The model under review builds one solid part; all positions refer to its coordinate system, in mm. A direction names the side the tool comes from. Coordinates: 2 decimals unless noted, no trailing zeros. Order: outer loops, then holes, each group sorted by start corner. A loop starts at its lowest first (then second) coordinate and runs counter-clockwise, first axis right, second up. Notation, with made-up numbers: (-8, 23) -> (15, 23) arc R17 ccw to (15, 39) -> close; hole circle Ø7 at (54.25, 4). An arc over 180 degrees is marked (long way). Use CSV: the item, a comma, the result in double quotes. Start each with the question number.
```python
from build123d import *

# Parameters (mm, degrees)
SKETCH1_R           = 1.1
SKETCH1_R_2         = 1.099999998
SKETCH1_R_3         = 1.100000002
SKETCH1_R_4         = 1.100000004
SKETCH1_R_5         = 1.099999996
SKETCH1_R_6         = 1.5
BOSS_EXTRUDE1_DEPTH = 3
SKETCH2_W           = 6.5
SKETCH2_H           = 3.5
CUT_EXTRUDE1_DEPTH  = 3


with BuildPart() as part:
    # Sketch1 → Boss-Extrude1 (new body)
    with BuildSketch(Plane(origin=(0, 0, 0), x_dir=(1, 0, 0), z_dir=(0, 1, 0))):
        with BuildLine():
            Line((-65.541413555, 48.16007559), (-33.218669872, 45.046086874))
            ThreePointArc((-33.218669872, 45.046086874), (-32.739740879, 45.011528364), (-32.25970508, 45))
            Line((-32.25970508, 45), (32.25970508, 45))
            ThreePointArc((32.25970508, 45), (32.739740879, 45.011528364), (33.218669872, 45.046086874))
            Line((33.218669872, 45.046086874), (65.541413555, 48.16007559))
            ThreePointArc((65.541413555, 48.16007559), (68.051615849, 48.735029299), (70.331753828, 49.931966272))
            ThreePointArc((70.331753828, 49.931966272), (81.716587017, 44.695249474), (71.540883348, 37.381380156))
            ThreePointArc((71.540883348, 37.381380156), (69.074176187, 38.121003778), (66.500378347, 38.206162463))
            Line((66.500378347, 38.206162463), (37.020517604, 35.366058461))
            ThreePointArc((37.020517604, 35.366058461), (34.967820887, 34.700490182), (33.386772404, 33.231874971))
            ThreePointArc((33.386772404, 33.231874971), (34.463229219, 29.741424145), (35.835420758, 26.3562954))
            ThreePointArc((35.835420758, 26.3562954), (35.77253489, 25.409347753), (34.946904251, 24.941374967))
            ThreePointArc((34.946904251, 24.941374967), (33.213559493, 24.190832889), (32.5, 22.441938863))
            Line((32.5, 22.441938863), (32.5, -22.441938863))
            ThreePointArc((32.5, -22.441938863), (33.213559493, -24.190832889), (34.946904251, -24.941374967))
            ThreePointArc((34.946904251, -24.941374967), (35.77253489, -25.409347753), (35.835420758, -26.3562954))
            ThreePointArc((35.835420758, -26.3562954), (34.463229219, -29.741424145), (33.386772404, -33.231874971))
            ThreePointArc((33.386772404, -33.231874971), (34.967820887, -34.700490182), (37.020517604, -35.366058461))
            Line((37.020517604, -35.366058461), (66.500378347, -38.206162463))
            ThreePointArc((66.500378347, -38.206162463), (69.074176187, -38.121003778), (71.540883348, -37.381380156))
            ThreePointArc((71.540883348, -37.381380156), (81.716587017, -44.695249474), (70.331753828, -49.931966272))
            ThreePointArc((70.331753828, -49.931966272), (68.051615849, -48.735029299), (65.541413555, -48.16007559))
            Line((65.541413555, -48.16007559), (33.218669872, -45.046086874))
            ThreePointArc((33.218669872, -45.046086874), (32.739740879, -45.011528364), (32.25970508, -45))
            Line((32.25970508, -45), (-32.25970508, -45))
            ThreePointArc((-32.25970508, -45), (-32.739740879, -45.011528364), (-33.218669872, -45.046086874))
            Line((-33.218669872, -45.046086874), (-65.541413555, -48.16007559))
            ThreePointArc((-65.541413555, -48.16007559), (-68.051615849, -48.735029299), (-70.331753828, -49.931966272))
            ThreePointArc((-70.331753828, -49.931966272), (-81.716587017, -44.695249474), (-71.540883348, -37.381380156))
            ThreePointArc((-71.540883348, -37.381380156), (-69.074176187, -38.121003778), (-66.500378347, -38.206162463))
            Line((-66.500378347, -38.206162463), (-37.020517604, -35.366058461))
            ThreePointArc((-37.020517604, -35.366058461), (-34.967820887, -34.700490182), (-33.386772404, -33.231874971))
            ThreePointArc((-33.386772404, -33.231874971), (-34.463229219, -29.741424145), (-35.835420758, -26.3562954))
            ThreePointArc((-35.835420758, -26.3562954), (-35.77253489, -25.409347753), (-34.946904251, -24.941374967))
            ThreePointArc((-34.946904251, -24.941374967), (-33.213559493, -24.190832889), (-32.5, -22.441938863))
            Line((-32.5, -22.441938863), (-32.5, 22.441938863))
            ThreePointArc((-32.5, 22.441938863), (-33.213559493, 24.190832889), (-34.946904251, 24.941374967))
            ThreePointArc((-34.946904251, 24.941374967), (-35.77253489, 25.409347753), (-35.835420758, 26.3562954))
            ThreePointArc((-35.835420758, 26.3562954), (-34.463229219, 29.741424145), (-33.386772404, 33.231874971))
            ThreePointArc((-33.386772404, 33.231874971), (-34.967820887, 34.700490182), (-37.020517604, 35.366058461))
            Line((-37.020517604, 35.366058461), (-66.500378347, 38.206162463))
            ThreePointArc((-66.500378347, 38.206162463), (-69.074176187, 38.121003778), (-71.540883348, 37.381380156))
            ThreePointArc((-71.540883348, 37.381380156), (-81.716587017, 44.695249474), (-70.331753828, 49.931966272))
            ThreePointArc((-70.331753828, 49.931966272), (-68.051615849, 48.735029299), (-65.541413555, 48.16007559))
        make_face()
        with Locations(Location((-79, 44, 0), (0, 0, 270))):
            Circle(SKETCH1_R, mode=Mode.SUBTRACT)
        with Locations(Location((79, 44, 0), (0, 0, 270))):
            Circle(SKETCH1_R, mode=Mode.SUBTRACT)
        with Locations(Location((-74.500002544, 48.500002544, 0), (0, 0, 270))):
            Circle(SKETCH1_R_2, mode=Mode.SUBTRACT)
        with Locations(Location((-70, 44.000005089, 0), (0, 0, 270))):
            Circle(SKETCH1_R_3, mode=Mode.SUBTRACT)
        with Locations(Location((-74.499997456, 39.500002544, 0), (0, 0, 270))):
            Circle(SKETCH1_R_4, mode=Mode.SUBTRACT)
        with Locations(Location((-74.499997456, -39.500002544, 0), (0, 0, 270))):
            Circle(SKETCH1_R_3, mode=Mode.SUBTRACT)
        with Locations(Location((-70, -44.000005089, 0), (0, 0, 270))):
            Circle(SKETCH1_R_2, mode=Mode.SUBTRACT)
        with Locations(Location((-74.500002544, -48.500002544, 0), (0, 0, 270))):
            Circle(SKETCH1_R_5, mode=Mode.SUBTRACT)
        with Locations(Location((-79, -44, 0), (0, 0, 270))):
            Circle(SKETCH1_R, mode=Mode.SUBTRACT)
        with Locations(Location((79, -44, 0), (0, 0, 270))):
            Circle(SKETCH1_R, mode=Mode.SUBTRACT)
        with Locations(Location((74.500002544, -48.500002544, 0), (0, 0, 270))):
            Circle(SKETCH1_R_3, mode=Mode.SUBTRACT)
        with Locations(Location((70, -44.000005089, 0), (0, 0, 270))):
            Circle(SKETCH1_R_2, mode=Mode.SUBTRACT)
        with Locations(Location((74.499997456, -39.500002544, 0), (0, 0, 270))):
            Circle(SKETCH1_R_5, mode=Mode.SUBTRACT)
        with Locations(Location((74.499997456, 39.500002544, 0), (0, 0, 270))):
            Circle(SKETCH1_R_2, mode=Mode.SUBTRACT)
        with Locations(Location((70, 44.000005089, 0), (0, 0, 270))):
            Circle(SKETCH1_R_3, mode=Mode.SUBTRACT)
        with Locations(Location((74.500002544, 48.500002544, 0), (0, 0, 270))):
            Circle(SKETCH1_R_4, mode=Mode.SUBTRACT)
        with Locations(Location((-74.5, -44, 0), (0, 0, 270))):
            Circle(SKETCH1_R_6, mode=Mode.SUBTRACT)
        with Locations(Location((-74.5, 44, 0), (0, 0, 270))):
            Circle(SKETCH1_R_6, mode=Mode.SUBTRACT)
        with Locations(Location((74.5, 44, 0), (0, 0, 270))):
            Circle(SKETCH1_R_6, mode=Mode.SUBTRACT)
        with Locations(Location((74.5, -44, 0), (0, 0, 270))):
            Circle(SKETCH1_R_6, mode=Mode.SUBTRACT)
    extrude(amount=BOSS_EXTRUDE1_DEPTH)

    # Sketch2 → Cut-Extrude1 (cut)
    with BuildSketch(Plane(origin=(0, 3, 0), x_dir=(1, 0, 0), z_dir=(0, 1, 0))):
        with Locations((-17.75, 23.75)):
            Rectangle(SKETCH2_W, SKETCH2_H)
        with Locations((-17.75, -23.75)):
            Rectangle(SKETCH2_W, SKETCH2_H)
        with Locations((17.75, -23.75)):
            Rectangle(SKETCH2_W, SKETCH2_H)
        with Locations((17.75, 23.75)):
            Rectangle(SKETCH2_W, SKETCH2_H)
        with BuildLine():
            Line((-25.5, 19), (-4, 19))
            ThreePointArc((-4, 19), (-3.292893219, 18.707106781), (-3, 18))
            Line((-3, 18), (-3, 2.5))
            ThreePointArc((-3, 2.5), (-3.292893219, 1.792893219), (-4, 1.5))
            Line((-4, 1.5), (-25.5, 1.5))
            ThreePointArc((-25.5, 1.5), (-26.207106781, 1.792893219), (-26.5, 2.5))
            Line((-26.5, 2.5), (-26.5, 18))
            ThreePointArc((-26.5, 18), (-26.207106781, 18.707106781), (-25.5, 19))
        make_face()
        with BuildLine():
            Line((-25.5, -1.5), (-4, -1.5))
            ThreePointArc((-4, -1.5), (-3.292893219, -1.792893219), (-3, -2.5))
            Line((-3, -2.5), (-3, -18))
            ThreePointArc((-3, -18), (-3.292893219, -18.707106781), (-4, -19))
            Line((-4, -19), (-25.5, -19))
            ThreePointArc((-25.5, -19), (-26.207106781, -18.707106781), (-26.5, -18))
            Line((-26.5, -18), (-26.5, -2.5))
            ThreePointArc((-26.5, -2.5), (-26.207106781, -1.792893219), (-25.5, -1.5))
        make_face()
        with BuildLine():
            Line((4, 19), (25.5, 19))
            ThreePointArc((25.5, 19), (26.207106781, 18.707106781), (26.5, 18))
            Line((26.5, 18), (26.5, 2.5))
            ThreePointArc((26.5, 2.5), (26.207106781, 1.792893219), (25.5, 1.5))
            Line((25.5, 1.5), (4, 1.5))
            ThreePointArc((4, 1.5), (3.292893219, 1.792893219), (3, 2.5))
            Line((3, 2.5), (3, 18))
            ThreePointArc((3, 18), (3.292893219, 18.707106781), (4, 19))
        make_face()
        with BuildLine():
            Line((4, -1.5), (25.5, -1.5))
            ThreePointArc((25.5, -1.5), (26.207106781, -1.792893219), (26.5, -2.5))
            Line((26.5, -2.5), (26.5, -18))
            ThreePointArc((26.5, -18), (26.207106781, -18.707106781), (25.5, -19))
            Line((25.5, -19), (4, -19))
            ThreePointArc((4, -19), (3.292893219, -18.707106781), (3, -18))
            Line((3, -18), (3, -2.5))
            ThreePointArc((3, -2.5), (3.292893219, -1.792893219), (4, -1.5))
        make_face()
        with BuildLine():
            Line((-17.595187003, 39), (17.595187003, 39))
            ThreePointArc((17.595187003, 39), (18.554660419, 38.281799152), (18.135944594, 37.158821525))
            Line((18.135944594, 37.158821525), (0.540757591, 25.84762988))
            ThreePointArc((0.540757591, 25.84762988), (0, 25.688808356), (-0.540757591, 25.84762988))
            Line((-0.540757591, 25.84762988), (-18.135944594, 37.158821525))
            ThreePointArc((-18.135944594, 37.158821525), (-18.554660419, 38.281799152), (-17.595187003, 39))
        make_face()
        with BuildLine():
            Line((-17.595187003, -39), (17.595187003, -39))
            ThreePointArc((17.595187003, -39), (18.554660419, -38.281799152), (18.135944594, -37.158821525))
            Line((18.135944594, -37.158821525), (0.540757591, -25.84762988))
            ThreePointArc((0.540757591, -25.84762988), (0, -25.688808356), (-0.540757591, -25.84762988))
            Line((-0.540757591, -25.84762988), (-18.135944594, -37.158821525))
            ThreePointArc((-18.135944594, -37.158821525), (-18.554660419, -38.281799152), (-17.595187003, -39))
        make_face()
    extrude(amount=-CUT_EXTRUDE1_DEPTH, mode=Mode.SUBTRACT)


solid = part.part
```
Q1. Add section C-C, the plane y = 1.55. State how many separate pieces and enclosed holes the cut face has, then the cut area to 3 significant figures.
Q2. Add section D-D, the plane x = 30. State the section outline as (y, z) points, then the cut area to 3 significant figures.
Q3. Clearance check with flat-ended pins moving along their axes: pin 1 Ø0.9 at (x, y) = (-16, 1) entering from +Z; pin 2 Ø1.5 at (x, y) = (-16.5, 1) entering from -Z; pin 3 Ø1 at (y, z) = (2.5, -14) entering from -X. State where each tip first meets the part, or that it passes through.
Q4. Add section A-A, the plane z = 8. State the section outline as (x, y) points.
Q5. For faces 1 (the cylindrical face through (34.994, 1.479, -34.716)), 2 (the flat face through (-3, 2, -10)), 3 (the flat face through (-49.606, 1.479, -46.625)), list the 3-axis set-ups (+Z, -Z, +X, -X, +Y, -Y) from which the entire face can be reached by the end or side of a thin tool; tool diameter is ignored.
Q6. Add section B-B, the plane z = 30. State the section outline as (x, y) points.
Q7. To check wall thickness, follow probe 1 along Z at (x, y) = (-21.5, 0.4); probe 2 along X at (y, z) = (2.9, -13); probe 3 along Z at (x, y) = (70, 1.9). State the ranges of each line that lie inside material, in increasing order.
Q8. Draft analysis for pull direction X (two halves, no side actions). For faces 4 (the flat face through (-18, 2, -25.5)), 5 (the flat face through (32.5, 1, 0)), 6 (the flat face through (0, 0, 4)), state which applies: +X half, -X half, draft (parallel to the pull), parting line (faces both ways), or undercut.
Answer block:
1,separate pieces,"1"
1,enclosed holes,"30"
1,area,"5,650 mm²"
2,outline,"(0, -45) -> (3, -45) -> (3, 45) -> (0, 45) -> close"
2,area,"270 mm²"
3,pin 1,"stops at z = 45"
3,pin 2,"stops at z = -45"
3,pin 3,"stops at x = -32.5"
4,outline,"(-32.5, 0) -> (-26.5, 0) -> (-26.5, 3) -> (-32.5, 3) -> close; (-3, 0) -> (3, 0) -> (3, 3) -> (-3, 3) -> close; (26.5, 0) -> (32.5, 0) -> (32.5, 3) -> (26.5, 3) -> close"
5,face 1,"+X, +Y, -Y"
5,face 2,"+Y, -Y"
5,face 3,"-Z, +Y, -Y"
6,outline,"(-34.37, 0) -> (-7, 0) -> (-7, 3) -> (-34.37, 3) -> close; (7, 0) -> (34.37, 0) -> (34.37, 3) -> (7, 3) -> close"
7,probe 1,"z = -45 to -19, -1.5 to 1.5, 19 to 45"
7,probe 2,"x = -32.5 to -26.5, -3 to 3, 26.5 to 32.5"
7,probe 3,"z = -49.71 to -45.1, -42.9 to -37.92, 37.92 to 42.9, 45.1 to 49.71"
8,face 4,"undercut"
8,face 5,"+X half"
8,face 6,"draft"
